Design review of the part shown in the three views and the two pictorial views. Dimensions are in mm from the part's minimum x, y and z. Coordinates: 2 decimals unless noted, no trailing zeros. Order: outer loops, then holes, each group sorted by start corner. A loop starts at its lowest first (then second) coordinate and runs counter-clockwise, first axis right, second up. Notation, with made-up numbers: (55, 84.5) - (60, 84.5) arc R22 cw to (60, 122.5) - close; hole circle Ø1 at (49.25, 48). An arc over 180 degrees is marked (long way). One line per item, written item: value. Start each with the question number.
(1) Mouldability with a two-part tool opening along Y and no side actions: class the marked faces 1, 2 and 3 as released by +Y, released by -Y, zero draft, split by the parting line, or undercut.
(2) Consider section A-A on z = 3.2. Write out the cut boundary in (x, y).
(3) Consider section D-D on z = 0.8. Write out the cut boundary in (x, y).
(4) Consider section B-B on y = 20.5. Write out the cut boundary in (x, z).
(5) To check wall thickness, follow line 1 along Y through (x, z) = (7.5, 0.95); line 2 along Z through (x, y) = (7.25, 16); line 3 along X through (y, z) = (20.75, 1.15). State the ranges of each line that lie inside material, in increasing order.
(6) Consider section C-C on x = 7.5. Write out the cut boundary in (y, z).
(7) Clearance check with flat-ended pins moving along their axes: pin 1 (1.3 mm diameter, centred on y = 9, z = 0.5, fed in from -X); pin 2 (2 mm diameter, centred on x = 9, y = 19.5, fed in from +Z); pin 3 (2 mm diameter, centred on y = 14, z = 2.5, fed in from +X); pin 4 (1.5 mm diameter, centred on x = 7.5, z = 3, fed in from +Y). State where each tip first meets the part, or that it passes through.
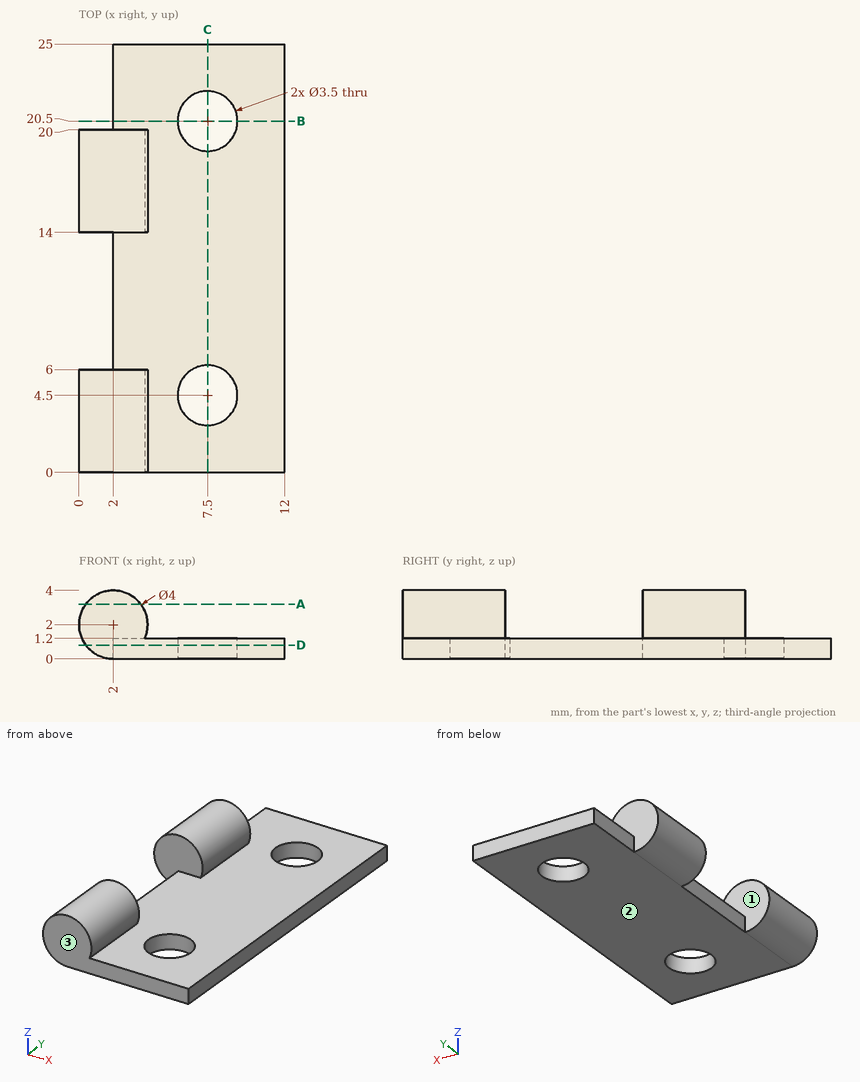
Geometry check:
1. face 1: undercut
1. face 2: zero draft
1. face 3: released by -Y
2. outline: (0.4, 0) - (3.6, 0) - (3.6, 6) - (0.4, 6) - close; (0.4, 14) - (3.6, 14) - (3.6, 20) - (0.4, 20) - close
3. outline: (0.4, 0) - (12, 0) - (12, 25) - (2, 25) - (2, 20) - (0.4, 20) - (0.4, 14) - (2, 14) - (2, 6) - (0.4, 6) - close; hole circle Ø3.5 at (7.5, 4.5); hole circle Ø3.5 at (7.5, 20.5)
4. outline: (2, 0) - (5.75, 0) - (5.75, 1.2) - (2, 1.2) - close; (9.25, 0) - (12, 0) - (12, 1.2) - (9.25, 1.2) - close
5. line 1: y = 0 to 2.75, 6.25 to 18.75, 22.25 to 25
5. line 2: z = 0 to 1.2
5. line 3: x = 2 to 5.77, 9.23 to 12
6. outline: (0, 0) - (2.75, 0) - (2.75, 1.2) - (0, 1.2) - close; (6.25, 0) - (18.75, 0) - (18.75, 1.2) - (6.25, 1.2) - close; (22.25, 0) - (25, 0) - (25, 1.2) - (22.25, 1.2) - close
7. pin 1: stops at x = 2
7. pin 2: stops at z = 1.2
7. pin 3: stops at x = 4
7. pin 4: passes through
